Geometry: final body of the model. Coordinates: model frame, mm. Face numbers are marked on the shaded views. A direction names the side the tool comes from. Give positions to 0.01 mm unless a question says otherwise; leave off trailing zeros. Write each loop counter-clockwise with the first axis right and the second up, starting at its lowest first coordinate (ties: lowest second). Pieces come first, ordered by that corner, then holes.
Q1. Reachability of the marked faces 1, 2, 3, 4 and 5 from +Z, -Z, +X, -X, +Y, -Y: full face, straight path, thin tool, end or side. Return the list, or none.
Q2. Cut plane A-A on x = -18. Return the cut outline in (y, z), plus the area to 3 significant figures.
Q3. Cut plane D-D on x = -7. Return the cut outline in (y, z), plus the area to 3 significant figures.
Q4. Cut plane C-C on y = -28. Return the cut outline in (x, z), plus the area to 3 significant figures.
Q5. Cut plane B-B on z = 3. Return the cut outline in (x, y).
Q6. Pin query (flat end, axial travel): pin 1 (6 mm diameter, centred on x = 15, y = -20.5, fed in from +Z); pin 2 (9 mm diameter, centred on x = 1, y = -7.5, fed in from +Z); pin 3 (5 mm diameter, centred on x = 17, z = 7, fed in from +Y). Return the tip coordinate at first contact, or that it passes through.
Q7. Line query: L1, parallel to Y at x = -18, z = 0.55; L2, parallel to X at y = -8, z = 5; L3, parallel to Z at x = -11.5, y = 13.5. Output: solid intervals per line, ascending.
```python
from build123d import *

# Parameters (mm, degrees)
SKETCH_W      = 40
SKETCH_H      = 60
PAD_DEPTH     = 1.5
SKETCH001_R   = 1
POCKET_DEPTH  = 1.501
SKETCH002_W   = 18
SKETCH002_H   = 43
PAD001_DEPTH  = 20
SKETCH003_W   = 7
SKETCH003_H   = 5
PAD002_DEPTH  = 10
SKETCH004_W   = 6
SKETCH004_H   = 12
SKETCH004_H_2 = 15
SKETCH004_H_3 = 7
PAD003_DEPTH  = 12


with BuildPart() as part:
    # Sketch → Pad (new body)
    with BuildSketch(Plane.XY):
        Rectangle(SKETCH_W, SKETCH_H)
    extrude(amount=PAD_DEPTH)

    # Sketch001 (on Face6 of Pad) → Pocket (cut, through all)
    with BuildSketch(Plane.XY.offset(1.5)):
        with Locations((-18, 28)):
            Circle(SKETCH001_R)
        with Locations((18, 28)):
            Circle(SKETCH001_R)
        with Locations((-18, -28)):
            Circle(SKETCH001_R)
        with Locations((18, -28)):
            Circle(SKETCH001_R)
    extrude(amount=-POCKET_DEPTH, mode=Mode.SUBTRACT)

    # Sketch002 (on Face5 of Pocket) → Pad001 (join)
    with BuildSketch(Plane.XY.offset(1.5)):
        with Locations((-1, -5.5)):
            Rectangle(SKETCH002_W, SKETCH002_H)
    extrude(amount=PAD001_DEPTH)

    # Sketch003 (on Face15 of Pad001) → Pad002 (join)
    with BuildSketch(Plane.XY.offset(21.5)):
        with Locations((-0.5, 13.5)):
            Rectangle(SKETCH003_W, SKETCH003_H)
    extrude(amount=PAD002_DEPTH)

    # Sketch004 (on Face5 of Pad002) → Pad003 (join)
    with BuildSketch(Plane.XY.offset(1.5)):
        with Locations((-16, -20)):
            Rectangle(SKETCH004_W, SKETCH004_H)
        with Locations((-16, -3.5)):
            Rectangle(SKETCH004_W, SKETCH004_H_2)
        with Locations((16, 22.5)):
            Rectangle(SKETCH004_W, SKETCH004_H_3)
    extrude(amount=PAD003_DEPTH)


solid = part.part
```
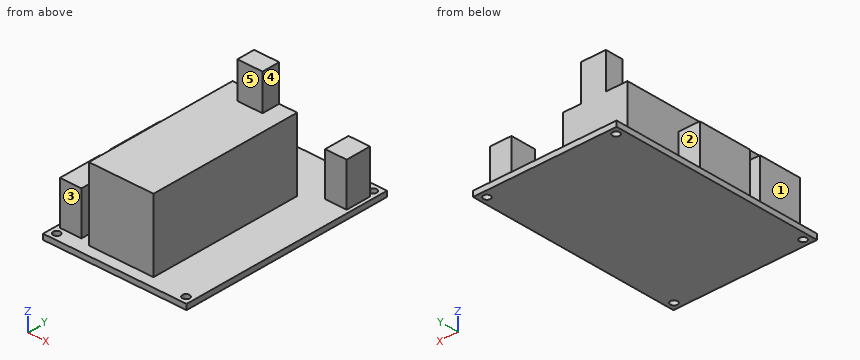
Data:
1. face 1: +Z, -X, +Y, -Y
1. face 2: +Z, -X, +Y
1. face 3: +Z, -X, -Y
1. face 4: +Z, +X, +Y, -Y
1. face 5: +Z, +X, -X, -Y
2. outline: (-30, 0) - (-29, 0) - (-29, 1.5) - (-30, 1.5) - close; (-27, 0) - (27, 0) - (27, 1.5) - (4, 1.5) - (4, 13.5) - (-11, 13.5) - (-11, 1.5) - (-14, 1.5) - (-14, 13.5) - (-26, 13.5) - (-26, 1.5) - (-27, 1.5) - close; (29, 0) - (30, 0) - (30, 1.5) - (29, 1.5) - close
2. area: 408 mm2
3. outline: (-30, 0) - (30, 0) - (30, 1.5) - (16, 1.5) - (16, 21.5) - (-27, 21.5) - (-27, 1.5) - (-30, 1.5) - close
3. area: 950 mm2
4. outline: (-20, 0) - (-19, 0) - (-19, 1.5) - (-20, 1.5) - close; (-17, 0) - (17, 0) - (17, 1.5) - (-17, 1.5) - close; (19, 0) - (20, 0) - (20, 1.5) - (19, 1.5) - close
4. area: 54.0 mm2
5. outline: (-19, -26) - (-13, -26) - (-13, -14) - (-19, -14) - close; (-19, -11) - (-13, -11) - (-13, 4) - (-19, 4) - close; (-10, -27) - (8, -27) - (8, 16) - (-10, 16) - close; (13, 19) - (19, 19) - (19, 26) - (13, 26) - close
6. pin 1: stops at z = 1.5
6. pin 2: stops at z = 21.5
6. pin 3: stops at y = 26
7. L1: y = -30 to -29, -27 to 27, 29 to 30
7. L2: x = -19 to -13, -10 to 8
7. L3: z = 0 to 1.5
